Build history of the part. All positions in model axes, mm. A direction names the side the tool comes from. Round coordinates to 2 decimals unless told otherwise and drop trailing zeros. Order: outer loops, then holes, each group sorted by start corner. A loop starts at its lowest first (then second) coordinate and runs counter-clockwise, first axis right, second up. Notation, with made-up numbers: M 78.25,-22.5 L 95.25,-22.5 A7 ccw 95.25,-11.5 Z; hole C 60.25,87 d9. An arc over 180 degrees is marked long. Use CSV: the item, a comma, the result in double quotes.
from build123d import *

# Parameters (mm, degrees)
BOSS_EXTRUDE1_DEPTH = 4.5
SKETCH3_R           = 10.5
CUT_EXTRUDE1_DEPTH  = 2
CUT_EXTRUDE2_REACH  = 6.5
SKETCH4_R           = 1.45


with BuildPart() as part:
    # Sketch2 → Boss-Extrude1 (new body)
    with BuildSketch(Plane.XY):
        with BuildLine():
            ThreePointArc((18.5, -7.599342077), (15, 0), (18.5, 7.599342077))
            ThreePointArc((18.5, 7.599342077), (18.47759065, 7.653668647), (18.455021767, 7.707929137))
            ThreePointArc((18.455021767, 7.707929137), (10.606601718, 10.606601718), (7.707929137, 18.455021767))
            ThreePointArc((7.707929137, 18.455021767), (7.653668647, 18.47759065), (7.599342077, 18.5))
            ThreePointArc((7.599342077, 18.5), (0, 15), (-7.599342077, 18.5))
            ThreePointArc((-7.599342077, 18.5), (-7.653668647, 18.47759065), (-7.707929137, 18.455021767))
            ThreePointArc((-7.707929137, 18.455021767), (-7.685237295, 18.066640012), (-7.67766953, 17.67766953))
            ThreePointArc((-7.67766953, 17.67766953), (-10.886996602, 10.33690927), (-18.455021767, 7.707929137))
            ThreePointArc((-18.455021767, 7.707929137), (-18.47759065, 7.653668647), (-18.5, 7.599342077))
            ThreePointArc((-18.5, 7.599342077), (-15.917048938, 4.183300133), (-15, 0))
            ThreePointArc((-15, 0), (-15.917048938, -4.183300133), (-18.5, -7.599342077))
            ThreePointArc((-18.5, -7.599342077), (-18.47759065, -7.653668647), (-18.455021767, -7.707929137))
            ThreePointArc((-18.455021767, -7.707929137), (-10.886996602, -10.33690927), (-7.67766953, -17.67766953))
            ThreePointArc((-7.67766953, -17.67766953), (-7.685237295, -18.066640012), (-7.707929137, -18.455021767))
            ThreePointArc((-7.707929137, -18.455021767), (-7.653668647, -18.47759065), (-7.599342077, -18.5))
            ThreePointArc((-7.599342077, -18.5), (0, -15), (7.599342077, -18.5))
            ThreePointArc((7.599342077, -18.5), (7.653668647, -18.47759065), (7.707929137, -18.455021767))
            ThreePointArc((7.707929137, -18.455021767), (10.606601718, -10.606601718), (18.455021767, -7.707929137))
            ThreePointArc((18.455021767, -7.707929137), (18.47759065, -7.653668647), (18.5, -7.599342077))
        make_face()
    extrude(amount=BOSS_EXTRUDE1_DEPTH)

    # Sketch3 → Cut-Extrude1 (cut)
    with BuildSketch(Plane.XY):
        Circle(SKETCH3_R)
    extrude(amount=CUT_EXTRUDE1_DEPTH, mode=Mode.SUBTRACT)

    # Sketch4 → Cut-Extrude2 (cut, up to next)
    with BuildSketch(Plane.XY.offset(4.5), mode=Mode.PRIVATE) as cut_extrude2_sk1:
        with Locations((0, 7)):
            Circle(SKETCH4_R)
    cut_extrude2_tool1 = extrude(cut_extrude2_sk1.sketch, amount=-CUT_EXTRUDE2_REACH, mode=Mode.PRIVATE) & part.part
    add(cut_extrude2_tool1.solids().sort_by_distance((0, 7, 4.5))[0], mode=Mode.SUBTRACT)
    # Sketch4 → Cut-Extrude2 (cut, up to next)
    with BuildSketch(Plane.XY.offset(4.5), mode=Mode.PRIVATE) as cut_extrude2_sk2:
        with Locations((7, 0)):
            Circle(SKETCH4_R)
    cut_extrude2_tool2 = extrude(cut_extrude2_sk2.sketch, amount=-CUT_EXTRUDE2_REACH, mode=Mode.PRIVATE) & part.part
    add(cut_extrude2_tool2.solids().sort_by_distance((7, 0, 4.5))[0], mode=Mode.SUBTRACT)
    # Sketch4 → Cut-Extrude2 (cut, up to next)
    with BuildSketch(Plane.XY.offset(4.5), mode=Mode.PRIVATE) as cut_extrude2_sk3:
        with Locations((0, -7)):
            Circle(SKETCH4_R)
    cut_extrude2_tool3 = extrude(cut_extrude2_sk3.sketch, amount=-CUT_EXTRUDE2_REACH, mode=Mode.PRIVATE) & part.part
    add(cut_extrude2_tool3.solids().sort_by_distance((0, -7, 4.5))[0], mode=Mode.SUBTRACT)
    # Sketch4 → Cut-Extrude2 (cut, up to next)
    with BuildSketch(Plane.XY.offset(4.5), mode=Mode.PRIVATE) as cut_extrude2_sk4:
        with Locations((-7, 0)):
            Circle(SKETCH4_R)
    cut_extrude2_tool4 = extrude(cut_extrude2_sk4.sketch, amount=-CUT_EXTRUDE2_REACH, mode=Mode.PRIVATE) & part.part
    add(cut_extrude2_tool4.solids().sort_by_distance((-7, 0, 4.5))[0], mode=Mode.SUBTRACT)


solid = part.part
(1) Tool access for faces 4 (the face through (0, 0, 2)), 5 (the face through (-0.314, -8.416, 3.268)): list every direction of +Z, -Z, +X, -X, +Y, -Y with a clear straight run to the whole face (end or side of a thin tool).
Answer block:
face 4,"-Z"
face 5,"+Z, -Z"
(2) Cut at B-B, the plane z = 0.45. Give the cut face in (x, y).
Answer block:
outline,"M -18.5,-7.6 A20 ccw -18.46,-7.71 A10 cw -7.71,-18.46 A20 ccw -7.6,-18.5 A10 cw 7.6,-18.5 A20 ccw 7.71,-18.46 A10 cw 18.46,-7.71 A20 ccw 18.5,-7.6 A10 cw 18.5,7.6 A20 ccw 18.46,7.71 A10 cw 7.71,18.46 A20 ccw 7.6,18.5 A10 cw -7.6,18.5 A20 ccw -7.71,18.46 A10 cw -18.46,7.71 A20 ccw -18.5,7.6 A10 cw Z; hole C 0,0 d21"
(3) Cut at A-A, the plane z = 3.5. Give the cut face in (x, y), and give its area (3 significant figures).
Answer block:
outline,"M -18.5,-7.6 A20 ccw -18.46,-7.71 A10 cw -7.71,-18.46 A20 ccw -7.6,-18.5 A10 cw 7.6,-18.5 A20 ccw 7.71,-18.46 A10 cw 18.46,-7.71 A20 ccw 18.5,-7.6 A10 cw 18.5,7.6 A20 ccw 18.46,7.71 A10 cw 7.71,18.46 A20 ccw 7.6,18.5 A10 cw -7.6,18.5 A20 ccw -7.71,18.46 A10 cw -18.46,7.71 A20 ccw -18.5,7.6 A10 cw Z; hole C -7,0 d2.9; hole C 0,-7 d2.9; hole C 0,7 d2.9; hole C 7,0 d2.9"
area,"812 mm²"
(4) Two-plate mould, pull along Y, no slides. Class faces 1 (the face through (0, -15, 2)), 2 (the face through (1, -11, 0)), 3 (the face through (15, 0, 2)): released by +Y, released by -Y, zero draft, split by the parting line, or undercut.
Answer block:
face 1,"released by -Y"
face 2,"zero draft"
face 3,"undercut"
(5) Drop flat-ended pins along their axis: pin 1 (1.5 mm diameter, centred on y = 13.5, z = 1.5, fed in from +X); pin 2 (1.5 mm diameter, centred on y = -14, z = 4, fed in from +X); pin 3 (1.7 mm diameter, centred on x = 7, y = 0, fed in from -Z); pin 4 (1.5 mm diameter, centred on y = 2.5, z = 3, fed in from -X). Give the stop position or say it passes through.
Answer block:
pin 1,"stops at x = 8.98"
pin 2,"stops at x = 8.71"
pin 3,"passes through"
pin 4,"stops at x = -15.54"
(6) Cut at D-D, the plane y = -1. Give the cut face in (x, z), and give its area (3 significant figures).
Answer block:
outline,"M -15.05,0 L -10.45,0 L -10.45,2 L -8.05,2 L -8.05,4.5 L -15.05,4.5 Z; M -5.95,2 L 5.95,2 L 5.95,4.5 L -5.95,4.5 Z; M 8.05,2 L 10.45,2 L 10.45,0 L 15.05,0 L 15.05,4.5 L 8.05,4.5 Z"
area,"83.1 mm²"
(7) Wall check: line 1 (Z direction, x = -6, y = 3); line 2 (X direction, y = -1, z = 3.8); line 3 (X direction, y = 16, z = 2.55). Give the ranges that are in metal, low to high. Write a range as from..to.
Answer block:
line 1,"z = 2..4.5"
line 2,"x = -15.05..-8.05, -5.95..5.95, 8.05..15.05"
line 3,"x = -7.82..-4.36, 4.36..7.82"
(8) Cut at C-C, the plane y = -7. Give the cut face in (x, z).
Answer block:
outline,"M -17.86,0 L -7.83,0 L -7.83,2 L -1.45,2 L -1.45,4.5 L -17.86,4.5 Z; M 1.45,2 L 7.83,2 L 7.83,0 L 17.86,0 L 17.86,4.5 L 1.45,4.5 Z"
